Geometry check sheet. Reference: the model listing, model coordinates, mm. Face numbers are marked on the shaded views. A direction names the side the tool comes from. Coordinates: 2 decimals unless noted, no trailing zeros. Loops run counter-clockwise (first coordinate to the right, second up) from the corner with the lowest first, then second, coordinate; pieces in that order, holes last.
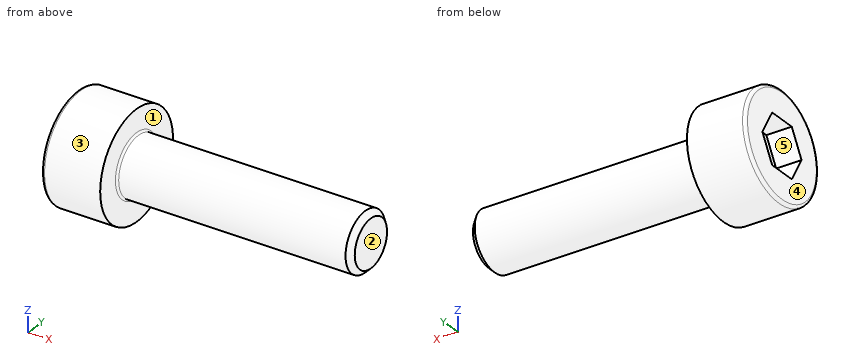
from build123d import *

# Parameters (mm, degrees)
CUT_EXTRUDE1_DEPTH = 1.3
FILLET1_R          = 0.15
CHAMFER1_SIZE      = 0.281
FILLET2_R          = 0.1


with BuildPart() as part:
    # Sketch1 → Revolve1 (revolve)
    with BuildSketch(Plane.XY, mode=Mode.PRIVATE) as revolve1_sk:
        Polygon((-3, 0), (-3, 2.75), (0, 2.75), (0, 1.5), (12, 1.5), (12, 0), align=None)
    revolve(revolve1_sk.sketch.rotate(Axis((0, 0, 0), (1, 0, 0)), 180), axis=Axis((0, 0, 0), (1, 0, 0)))

    # Sketch2 → Cut-Extrude1 (cut)
    with BuildSketch(Plane.ZY.offset(3)):
        Polygon((0, 1.478016689), (-1.28, 0.739008345), (-1.28, -0.739008345), (0, -1.478016689), (1.28, -0.739008345), (1.28, 0.739008345), align=None)
    extrude(amount=-CUT_EXTRUDE1_DEPTH, mode=Mode.SUBTRACT)

    # Fillet1
    fillet1_edges = [part.edges().sort_by_distance(p)[0] for p in [
        (-3, 2.75, 0),
    ]]
    fillet(fillet1_edges, radius=FILLET1_R)

    # Chamfer1
    chamfer1_edges = [part.edges().sort_by_distance(p)[0] for p in [
        (12, 1.5, 0),
    ]]
    chamfer(chamfer1_edges, length=CHAMFER1_SIZE)

    # Fillet2
    fillet2_edges = [part.edges().sort_by_distance(p)[0] for p in [
        (0, 1.5, 0),
    ]]
    fillet(fillet2_edges, radius=FILLET2_R)


solid = part.part
(1) Gauge pin test, flat ends, axial feed: pin 1 Ø1.3 at (y, z) = (0, -0.5) entering from -X; pin 2 Ø3 at (x, z) = (9, 0) entering from +Y. Record the tip position at first contact, or that the pin passes through.
Findings:
pin 1: stops at x = -1.7
pin 2: stops at y = 1.5
(2) Sectioned sample at C-C on x = 8. Record the cut outline in (y, z), and give its area (3 significant figures).
Findings:
outline: circle Ø3 at (0, 0)
area: 7.07 mm2
(3) Scan lines: L1, parallel to X at y = -1.5, z = 0.5; L2, parallel to X at y = 0.4, z = 1.1; L3, parallel to Z at x = 7.25, y = 0.1. Record each from-to range of solid material in increasing order.
Findings:
L1: x = -3 to 0
L2: x = -1.7 to 12
L3: z = -1.5 to 1.5
(4) Access from +Z, -Z, +X, -X, +Y, -Y to the whole of each face (thin tool, end or side, straight path). Record for the marked faces 1 and 2.
Findings:
face 1: +X
face 2: +Z, -Z, +X, +Y, -Y
(5) Draft check along Y on the marked faces 3, 4 and 5. Enter one of: +Y half, -Y half, draft (parallel to the pull), parting line (faces both ways), or undercut.
Findings:
face 3: parting line
face 4: draft
face 5: undercut
(6) Sectioned sample at B-B on x = -1.5. Record the cut outline in (y, z), and give its area (3 significant figures).
Findings:
outline: circle Ø5.5 at (0, 0)
area: 23.8 mm2
(7) Sectioned sample at A-A on y = 0. Record the cut outline in (x, z).
Findings:
outline: (-3, -2.6) arc R0.15 ccw to (-2.85, -2.75) - (0, -2.75) - (0, -1.6) arc R0.1 cw to (0.1, -1.5) - (11.72, -1.5) - (12, -1.22) - (12, 1.22) - (11.72, 1.5) - (0.1, 1.5) arc R0.1 cw to (0, 1.6) - (0, 2.75) - (-2.85, 2.75) arc R0.15 ccw to (-3, 2.6) - (-3, 1.28) - (-1.7, 1.28) - (-1.7, -1.28) - (-3, -1.28) - close
